The listing builds one solid part. Answer for the finished solid, in the listing's coordinates (mm). Face numbers are marked on the shaded views. A direction names the side the tool comes from. Give positions to 0.01 mm unless a question says otherwise; leave off trailing zeros. Order: outer loops, then holes, each group sorted by start corner. A loop starts at its lowest first (then second) coordinate and runs counter-clockwise, first axis right, second up. Notation, with made-up numbers: (70.5, -4) - (108.5, -4) arc R12 cw to (108.5, 16) - close; hole circle Ø4 at (4, 67.5). An arc over 180 degrees is marked (long way). Write each question's results on one line, items separated by ' | '. Start each with the question number.
1. Section D-D (x = -2) is taken. Give the vertices of the cut face in (y, z), and give its area (3 significant figures).
2. Section B-B (z = 5.25) is taken. Give the vertices of the cut face in (x, y), and give its area (3 significant figures).
3. Section A-A (x = 4) is taken. Give the vertices of the cut face in (y, z) (3 decimals), and give its area (3 significant figures).
4. Which of the six approach directions +Z, -Z, +X, -X, +Y, -Y give full straight-line access (tool end or side, diameter ignored) to the marked faces 5, 6 and 7?
5. Find the intervals of material crossed by L1, parallel to Y at x = -0.5, z = 2.75; L2, parallel to Y at x = 9, z = 4.5; L3, parallel to Y at x = 6, z = 1.75, in increasing order.
6. Flat-ended cylindrical pins translate along their axes: pin 1 (3 mm diameter, centred on y = 18.5, z = 3, fed in from -X); pin 2 (3 mm diameter, centred on y = 19, z = 2, fed in from +X); pin 3 (3 mm diameter, centred on x = 16, z = 4, fed in from +Y). Find the tip coordinate at first contact, or state that the pin passes through.
7. Determine the mould class of the marked faces 1, 2, 3 and 4 for opening direction Y: released by +Y, released by -Y, zero draft, split by the parting line, or undercut.
8. Section C-C (y = 17) is taken. Give the vertices of the cut face in (x, z), and give its area (3 significant figures).
from build123d import *

# Parameters (mm, degrees)
F1_DEPTH = 6.35
F3_D     = 1.778
F5_D     = 2.4384
F5_DEPTH = 5.08
F5_TIP   = 0.7325692667
F7_D     = 2.4384
F7_DEPTH = 25.4
F7_START = 7.3375843
F7_TIP   = 0.7325692667


with BuildPart() as f1:
    # F0 (on Top) → F1 (new body)
    with BuildSketch(Plane.XY):
        with BuildLine():
            Line((0, 14.708516188), (-11.6383890907, 14.708516188))
            Line((-11.6383890907, 14.708516188), (-11.6383890907, -28.471483812))
            Line((-11.6383890907, -28.471483812), (23.9216109093, -28.471483812))
            Line((23.9216109093, -28.471483812), (23.9216109093, 14.708516188))
            Line((23.9216109093, 14.708516188), (12.2091952547, 14.708516188))
            Line((12.2091952547, 14.708516188), (12.2091952547, 24.868516188))
            Line((12.2091952547, 24.868516188), (7.4116109093, 24.868516188))
            Line((7.4116109093, 24.868516188), (7.4116109093, 20.296516188))
            ThreePointArc((7.4116109093, 20.296516188), (6.1416109093, 13.946516188), (4.8716109093, 20.296516188))
            Line((4.8716109093, 20.296516188), (4.8716109093, 24.868516188))
            Line((4.8716109093, 24.868516188), (0, 24.868516188))
            Line((0, 24.868516188), (0, 14.708516188))
        make_face()
    extrude(amount=F1_DEPTH)

    # F3 (through all)
    with Locations(Plane.XY.offset(6.35)):
        with Locations((-7.8283890907, -5.611483812), (20.1116109093, -5.611483812), (20.1116109093, -18.311483812), (-7.8283890907, -18.311483812)):
            Hole(F3_D / 2)

    # F5
    with Locations(Plane.YZ.offset(12.2091952547)):
        with Locations((22.506316188, 3.175)):
            Hole(F5_D / 2, depth=F5_DEPTH)
            with Locations((0, 0, -(F5_DEPTH + F5_TIP / 2))):  # 118° drill point
                Cone(0, F5_D / 2, F5_TIP, mode=Mode.SUBTRACT)

    # F7
    # its depths count from where the whole tool has entered the part; down to there all is cleared
    with Locations(Plane.YZ.offset(12.2091952547).offset(-F7_START)):
        with Locations((22.519016188, 3.175)):
            Hole(F7_D / 2, depth=F7_DEPTH)
            with Locations((0, 0, -(F7_DEPTH + F7_TIP / 2))):  # 118° drill point
                Cone(0, F7_D / 2, F7_TIP, mode=Mode.SUBTRACT)


solid = f1.part
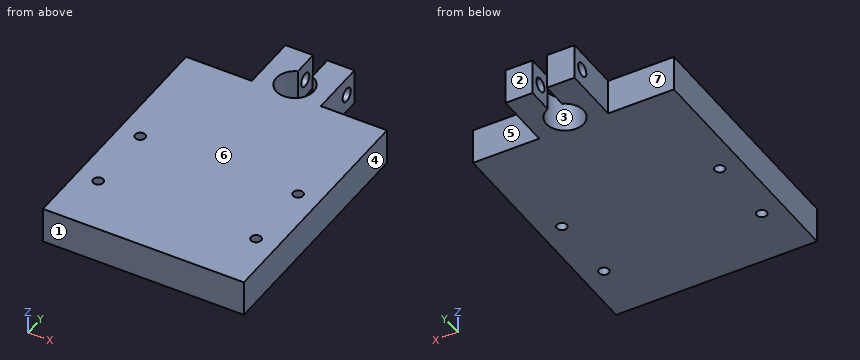
Reported:
1) outline: (-28.47, 0) - (14.71, 0) - (14.71, 6.35) - (-28.47, 6.35) - close | area: 274 mm²
2) outline: (-11.64, -28.47) - (23.92, -28.47) - (23.92, 14.71) - (12.21, 14.71) - (12.21, 24.87) - (7.41, 24.87) - (7.41, 20.3) arc R3.3 cw (long way) to (4.87, 20.3) - (4.87, 24.87) - (0, 24.87) - (0, 14.71) - (-11.64, 14.71) - close; hole circle Ø1.78 at (-7.83, -18.31); hole circle Ø1.78 at (-7.83, -5.61); hole circle Ø1.78 at (20.11, -18.31); hole circle Ø1.78 at (20.11, -5.61) | area: 1,600 mm²
3) outline: (-28.471, 0) - (14.735, 0) - (14.735, 6.35) - (-28.471, 6.35) - close; (19.762, 0) - (24.869, 0) - (24.869, 6.35) - (19.762, 6.35) - close; hole circle Ø2.438 at (22.519, 3.175) | area: 302 mm²
4) face 5: +Z, -Z, +X, +Y | face 6: +Z, +X, -X, +Y, -Y | face 7: +Z, -Z, -X, +Y
5) L1: -28.47 to 14.71 | L2: -28.47 to 15.6, 18.9 to 24.87 | L3: -28.47 to 13.95
6) pin 1: x = 0 | pin 2: x = 12.21 | pin 3: y = 14.71
7) face 1: released by -Y | face 2: released by +Y | face 3: undercut | face 4: zero draft
8) outline: (0, 0) - (2.85, 0) - (2.85, 6.35) - (0, 6.35) - close; (9.43, 0) - (12.21, 0) - (12.21, 6.35) - (9.43, 6.35) - close | area: 35.7 mm²
